Build history of the part. All positions in model axes, mm. Face numbers are marked on the shaded views. A direction names the side the tool comes from. Give positions to 0.01 mm unless a question says otherwise; leave off trailing zeros. Loops run counter-clockwise (first coordinate to the right, second up) from the corner with the lowest first, then second, coordinate; pieces in that order, holes last. Notation, with made-up numbers: (54.25, 25.5) - (109.25, 25.5) arc R19 cw to (109.25, 34.5) - close; hole circle Ø5 at (79.25, 76.5). An arc over 180 degrees is marked (long way). Return JSON: item names as keys, results as strings. Group by question number.
1) 3-axis set-ups, long thin cutter, end or side, ignore diameter. For the marked faces 5, 6, 7 and 8: which of +Z, -Z, +X, -X, +Y, -Y reach the whole face in a straight line?
2) Drill centre lines: probe 1 along X at (y, z) = (16.5, 1.5); probe 2 along X at (y, z) = (6.5, 4); probe 3 along Z at (x, y) = (8.25, 5.5). Where is each one in solid material? Low to high. Write a range as from..to.
3) Slice it at A-A (y = 17). List the corners of the cut face in (x, z), and give its area (3 significant figures).
4) Slice it at D-D (x = 17.5). List the corners of the cut face in (y, z).
5) Slice it at B-B (x = 10). List the corners of the cut face in (y, z).
6) Slice it at C-C (y = 25). List the corners of the cut face in (x, z).
7) Drop flat-ended pins along their axis: pin 1 (3.5 mm diameter, centred on x = 18, z = 25, fed in from +Y); pin 2 (4 mm diameter, centred on x = 13, z = 21.5, fed in from +Y); pin 3 (0.9 mm diameter, centred on x = 1.5, y = 26.5, fed in from +Z). Give the stop position or say it passes through.
8) Mould opens along X. For the marked faces 1, 2, 3 and 4 say: released by +X, released by -X, zero draft, split by the parting line, or undercut.
Autodesk Inventor part; units mm, degrees
ref_plane "Work Plane1" through (17, 0, 0) normal (1, 0, 0) x (0, 1, 0)
ref_plane "XZ Plane" through (0, 0, 0) normal (0, 1, 0) x (-1, 0, 0)
ref_plane "XY Plane" through (0, 0, 0) normal (0, 0, 1) x (1, 0, 0)
sketch "Sketch1" plane through (0, 0, 0) normal (1, 0, 0) x (0, 1, 0)
  line L0 (28, 5) -> (28, 0)
  line L1 (5, 23) -> (23, 5)
  line L2 (5, 28) -> (5, 23)
  line L3 (0, 0) -> (0, 28)
  line L4 (23, 5) -> (28, 5)
  line L5 (0, 28) -> (5, 28)
  line L6 (28, 0) -> (0, 0)
extrude "Extrusion4" add sketch "Sketch1" along normal blind 20
ref_plane "Work Plane1" through (17, 0, 0) normal (1, 0, 0) x (0, 1, 0)
sketch "Sketch2" plane through (17, 0, 0) normal (1, 0, 0) x (0, 1, 0)
  line L0 (3, 28) -> (3, 3)
  line L1 (5, 23) -> (23, 5)
  line L2 (3, 28) -> (5, 28)
  line L3 (23, 5) -> (28, 5)
  line L4 (3, 3) -> (28, 3)
  line L5 (5, 28) -> (5, 23)
  line L6 (28, 5) -> (28, 3)
extrude "Extrusion3" cut sketch "Sketch2" against normal blind 14
sketch "Sketch3" plane through (17, 3, 28) normal (0, 1, 0) x (1, 0, 0)
  arc A0 (-10, 9.5) -> (-4, 9.5) centre (-7, 9.5) ccw
  line L0 (-10, 9.5) -> (-10, 15.5)
  arc A1 (-4, 15.5) -> (-10, 15.5) centre (-7, 15.5) ccw
  line L1 (-4, 15.5) -> (-4, 9.5)
extrude "Extrusion2" cut sketch "Sketch3" against normal blind 3
sketch "Sketch4" plane through (0, 0, 0) normal (0, 0, 1) x (1, 0, 0)
  arc A0 (13, 18.5) -> (7, 18.5) centre (10, 18.5) ccw
  arc A1 (7, 12.5) -> (13, 12.5) centre (10, 12.5) ccw
  line L0 (13, 12.5) -> (13, 18.5)
  line L1 (7, 18.5) -> (7, 12.5)
extrude "Extrusion1" cut sketch "Sketch4" along normal blind 3 draft 0
properties part number "Corner Connector"
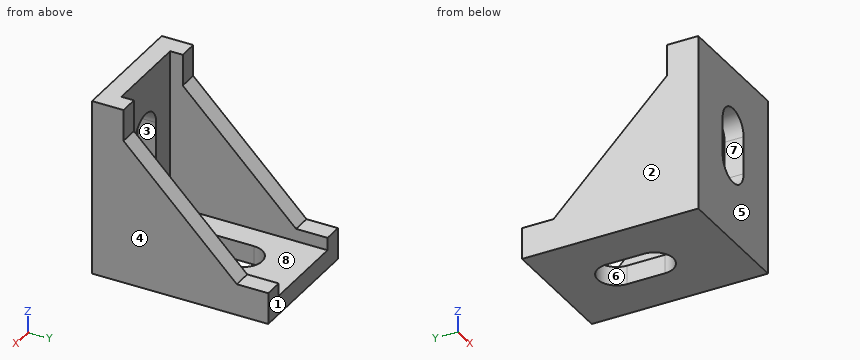
Results:
{
 "1": {"face 5": "+Z, -Z, +X, -X, -Y", "face 6": "+Z, -Z", "face 7": "+Y, -Y", "face 8": "+Z, +Y"},
 "2": {"probe 1": "0..7, 13..20", "probe 2": "0..3, 17..20", "probe 3": "0..3"},
 "3": {"outline": "(0, 0) - (7, 0) - (7, 3) - (3, 3) - (3, 11) - (0, 11) - close; (13, 0) - (20, 0) - (20, 11) - (17, 11) - (17, 3) - (13, 3) - close", "area": "90.0 mm2"},
 "4": {"outline": "(0, 0) - (28, 0) - (28, 5) - (23, 5) - (5, 23) - (5, 28) - (0, 28) - close"},
 "5": {"outline": "(0, 0) - (9.5, 0) - (9.5, 3) - (3, 3) - (3, 9.5) - (0, 9.5) - close; (0, 21.5) - (3, 21.5) - (3, 28) - (0, 28) - close; (21.5, 0) - (28, 0) - (28, 3) - (21.5, 3) - close"},
 "6": {"outline": "(0, 0) - (20, 0) - (20, 5) - (17, 5) - (17, 3) - (3, 3) - (3, 5) - (0, 5) - close"},
 "7": {"pin 1": "y = 5", "pin 2": "y = 3", "pin 3": "z = 5"},
 "8": {"face 1": "zero draft", "face 2": "released by -X", "face 3": "undercut", "face 4": "released by +X"}
}
